Source: CAD feature listing. Evaluate the final solid. Frame: model axes, mm. Face numbers are marked on the shaded views. A direction names the side the tool comes from. Coordinates: 2 decimals unless noted, no trailing zeros. Order: outer loops, then holes, each group sorted by start corner. A loop starts at its lowest first (then second) coordinate and runs counter-clockwise, first axis right, second up.
```python
from build123d import *

# Parameters (mm, degrees)
CYLINDER057_R     = 2
CYLINDER057_DEPTH = 13
CYLINDER059_R     = 3.25
CYLINDER059_DEPTH = 2.6
BOX019_W          = 6
BOX019_H          = 1.5
BOX019_DEPTH      = 14
ARRAY004_COUNT    = 8
CYLINDER055_R     = 10.5
CYLINDER055_DEPTH = 14


with BuildPart() as cylinder052:
    # Cylinder057 → Cylinder057 (new body)
    with BuildSketch(Plane.XY.offset(3.6)):
        Circle(CYLINDER057_R)
    extrude(amount=CYLINDER057_DEPTH)


with BuildPart() as cylinder054:
    # Cylinder059 → Cylinder059 (new body)
    with BuildSketch(Plane.XY.offset(1)):
        Circle(CYLINDER059_R)
    extrude(amount=CYLINDER059_DEPTH)


with BuildPart() as array004:
    # Box019 → Box019 (new body)
    with BuildSketch(Plane(origin=(6, -0.75, 0), x_dir=(1, 0, 0), z_dir=(0, 0, 1))):
        with Locations((3, 0.75)):
            Rectangle(BOX019_W, BOX019_H)
    extrude(amount=BOX019_DEPTH)

    # Array004: Array004 ×8 about axis
    array004_axis = Axis((0, 0, 0), (0, 0, 1))


with BuildPart() as array004_1:
    add(array004.part)
    for i in range(1, ARRAY004_COUNT):
        add(array004.part.rotate(array004_axis, i * 360 / ARRAY004_COUNT))


with BuildPart() as obj1:
    # Cylinder055 → Cylinder055 (new body)
    with BuildSketch(Plane.XY):
        Circle(CYLINDER055_R)
    extrude(amount=CYLINDER055_DEPTH)

    # Fusion021: union Array004
    add(array004_1.part)


with BuildPart() as obj1_1:
    # Fusion021 placement: moved
    add(obj1.part.moved(Location((0, 0, 1))))

    # Cut043: cut Cylinder054
    add(cylinder054.part, mode=Mode.SUBTRACT)

    # Cut044: cut Cylinder052
    add(cylinder052.part, mode=Mode.SUBTRACT)


solid = obj1_1.part
```
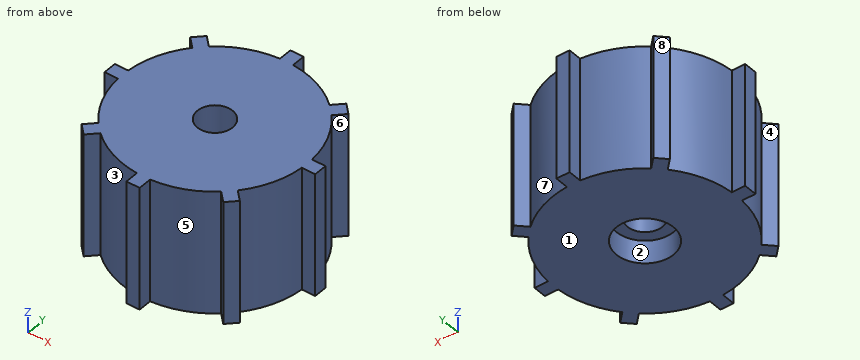
1. Access query for the marked faces 4, 5, 6, 7 and 8. Directions: +Z, -Z, +X, -X, +Y, -Y. A direction counts if a zero-diameter tool reaches every point of the face in a straight line with its end or side. Return the directions, or none.
Findings:
face 4: +Z, -Z, -X
face 5: +Z, -Z, -Y
face 6: +Z, -Z, +X
face 7: +Z, -Z, +Y
face 8: +Z, -Z, -X, +Y
2. Draft query along Y for the marked faces 1, 2 and 3. Return one class per face: released by +Y, released by -Y, zero draft, split by the parting line, or undercut.
Findings:
face 1: zero draft
face 2: undercut
face 3: released by -Y
3. Section query A-A on y = 0. Return loops of the section in (x, z), plus the area to 4 significant figures.
Findings:
outline: (-12, 1) - (-3.25, 1) - (-3.25, 3.6) - (-2, 3.6) - (-2, 15) - (-12, 15) - close; (2, 3.6) - (3.25, 3.6) - (3.25, 1) - (12, 1) - (12, 15) - (2, 15) - close
area: 273.5 mm2
4. Ray query, line 1 (Y direction, x = 0, z = 9); line 2 (Y direction, x = 0, z = 3). Return the intervals inside material, ascending.
Findings:
line 1: y = -12 to -2, 2 to 12
line 2: y = -12 to -3.25, 3.25 to 12
5. Section query D-D on x = -8.25. Return loops of the section in (y, z), plus the area to 3 significant figures.
Findings:
outline: (-8.72, 1) - (-7.19, 1) - (-7.19, 15) - (-8.72, 15) - close; (-6.5, 1) - (6.5, 1) - (6.5, 15) - (-6.5, 15) - close; (7.19, 1) - (8.72, 1) - (8.72, 15) - (7.19, 15) - close
area: 225 mm2
6. Pin query (flat end, axial travel): P1, Ø2, axis at y = -3, z = 13.5, coming from the -X side; P2, Ø6, axis at y = -4, z = 3.5, coming from the -X side; P3, Ø0.8, axis at x = 11, z = 5.5, coming from the -Y side; P4, Ø6, axis at x = 0, y = 0, coming from the +Z side. Return the tip coordinate at first contact, or that it passes through.
Findings:
P1: stops at x = -10.31
P2: stops at x = -10.45
P3: stops at y = -0.75
P4: stops at z = 15
